Check sheet for the modelled part. Datum: model origin and axes. Units: mm. Face numbers are marked on the shaded views. A direction names the side the tool comes from. Coordinates: 2 decimals unless noted, no trailing zeros. Write each loop counter-clockwise with the first axis right and the second up, starting at its lowest first coordinate (ties: lowest second). Pieces come first, ordered by that corner, then holes. Notation, with made-up numbers: (32, 29) -> (85, 29) arc R29 ccw to (85, 62) -> close; hole circle Ø7 at (52.5, 27). An arc over 180 degrees is marked (long way). One line per item, written item: value. Start each with the question number.
1) Scan lines: line 1 along Z through (x, y) = (0, -14.5); line 2 along Z through (x, y) = (0, 36); line 3 along Y through (x, z) = (-66, -20). Record each from-to range of solid material in increasing order. Write a range as [from, to].
2) Draft check along X on the marked faces 1, 2 and 3. Enter one of: +X half, -X half, draft (parallel to the pull), parting line (faces both ways), or undercut.
3) Gauge pin test, flat ends, axial feed: P1, Ø8, axis at y = -16.5, z = 54, coming from the +X side; P2, Ø1.5, axis at x = -56, z = -16, coming from the -Y side; P3, Ø19, axis at x = 21, y = -14.5, coming from the -Z side. Record the tip position at first contact, or that the pin passes through.
4) Set-up check for the marked faces 4, 5 and 6: record each of +Z, -Z, +X, -X, +Y, -Y from which the full face is reachable in a straight line by a thin tool's end or side.
5) Sectioned sample at A-A on x = 0. Enter the section's corners in (y, z).
6) Sectioned sample at D-D on z = -35. Enter the section's corners in (x, y), plus the area to 3 significant figures.
7) Sectioned sample at B-B on z = 0. Enter the section's corners in (x, y), plus the area to 3 significant figures.
8) Sectioned sample at C-C on y = 15.5. Enter the section's corners in (x, z), plus the area to 3 significant figures.
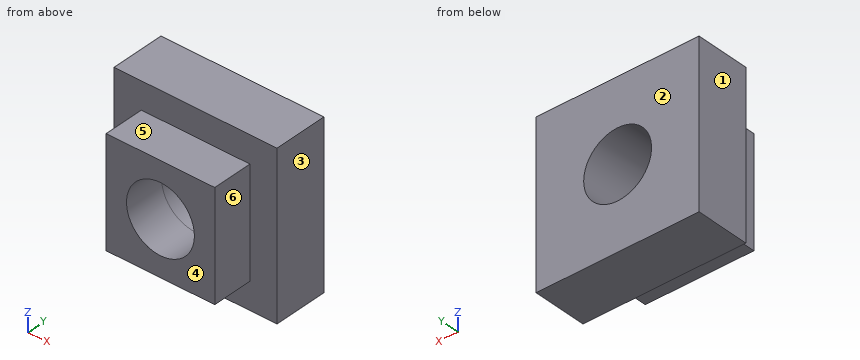
```python
from build123d import *

# Parameters (mm, degrees)
F0_W     = 101.6
F0_H     = 101.6
F0_R     = 31.75
F1_DEPTH = 38.1
F0_W_2   = 152.4
F0_H_2   = 152.4
F2_DEPTH = 50.8


with BuildPart() as f1:
    # F0 (on Front) → F1 (new body)
    with BuildSketch(Plane.XZ):
        Rectangle(F0_W, F0_H)
        Circle(F0_R, mode=Mode.SUBTRACT)
    extrude(amount=F1_DEPTH)

    # F0 (on Front) → F2 (join)
    with BuildSketch(Plane.XZ):
        Rectangle(F0_W_2, F0_H_2)
        Rectangle(F0_W, F0_H, mode=Mode.SUBTRACT)
        Rectangle(F0_W, F0_H)
        Circle(F0_R, mode=Mode.SUBTRACT)
    extrude(amount=-F2_DEPTH)


solid = f1.part
```
Answers:
1. line 1: z = [-50.8, -31.75], [31.75, 50.8]
1. line 2: z = [-76.2, -31.75], [31.75, 76.2]
1. line 3: y = [0, 50.8]
2. face 1: -X half
2. face 2: draft
2. face 3: +X half
3. P1: stops at x = 50.8
3. P2: stops at y = 0
3. P3: stops at z = -50.8
4. face 4: +Z, -Z, +X, -X, -Y
4. face 5: +Z, +X, -X, -Y
4. face 6: +Z, -Z, +X, -Y
5. outline: (-38.1, -50.8) -> (0, -50.8) -> (0, -76.2) -> (50.8, -76.2) -> (50.8, -31.75) -> (-38.1, -31.75) -> close; (-38.1, 31.75) -> (50.8, 31.75) -> (50.8, 76.2) -> (0, 76.2) -> (0, 50.8) -> (-38.1, 50.8) -> close
6. outline: (-76.2, 0) -> (-50.8, 0) -> (-50.8, -38.1) -> (50.8, -38.1) -> (50.8, 0) -> (76.2, 0) -> (76.2, 50.8) -> (-76.2, 50.8) -> close
6. area: 11,600 mm2
7. outline: (-76.2, 0) -> (-50.8, 0) -> (-50.8, -38.1) -> (-31.75, -38.1) -> (-31.75, 50.8) -> (-76.2, 50.8) -> close; (31.75, -38.1) -> (50.8, -38.1) -> (50.8, 0) -> (76.2, 0) -> (76.2, 50.8) -> (31.75, 50.8) -> close
7. area: 5,970 mm2
8. outline: (-76.2, -76.2) -> (76.2, -76.2) -> (76.2, 76.2) -> (-76.2, 76.2) -> close; hole circle Ø63.5 at (0, 0)
8. area: 20,100 mm2
